Can you work these out from the model? Positions are in its coordinate system, mm. Face numbers are marked on the shaded views. A direction names the side the tool comes from. Coordinates: 2 decimals unless noted, no trailing zeros. Loops run counter-clockwise (first coordinate to the right, second up) from the corner with the lowest first, then second, coordinate; pieces in that order, holes last.
```python
from build123d import *

# Parameters (mm, degrees)
SKETCH2_W           = 80
SKETCH2_H           = 100
BOSS_EXTRUDE1_DEPTH = 10
SKETCH3_W           = 20
SKETCH3_H           = 100
BOSS_EXTRUDE2_DEPTH = 120
SKETCH5_R           = 2.555
CUT_EXTRUDE2_DEPTH  = 55
SKETCH4_R           = 15
CUT_EXTRUDE3_DEPTH  = 29


with BuildPart() as part:
    # Sketch2 → Boss-Extrude1 (new body)
    with BuildSketch(Plane(origin=(0, 0, 0), x_dir=(1, 0, 0), z_dir=(0, 1, 0))):
        Rectangle(SKETCH2_W, SKETCH2_H)
    extrude(amount=BOSS_EXTRUDE1_DEPTH)

    # Sketch3 → Boss-Extrude2 (add)
    with BuildSketch(Plane(origin=(0, 10, 0), x_dir=(1, 0, 0), z_dir=(0, 1, 0))):
        Rectangle(SKETCH3_W, SKETCH3_H)
    extrude(amount=BOSS_EXTRUDE2_DEPTH)

    # Sketch5 → Cut-Extrude2 (cut)
    with BuildSketch(Plane.XZ):
        with Locations((-25.4, -38.1)):
            Circle(SKETCH5_R)
        with Locations((25.4, -38.1)):
            Circle(SKETCH5_R)
        with Locations((-25.4, 38.1)):
            Circle(SKETCH5_R)
        with Locations((25.4, 38.1)):
            Circle(SKETCH5_R)
    extrude(amount=-CUT_EXTRUDE2_DEPTH, mode=Mode.SUBTRACT)

    # Sketch4 → Cut-Extrude3 (cut)
    with BuildSketch(Plane.ZY.offset(10)):
        with Locations((0, 103.69)):
            Circle(SKETCH4_R)
    extrude(amount=-CUT_EXTRUDE3_DEPTH, mode=Mode.SUBTRACT)


solid = part.part
```
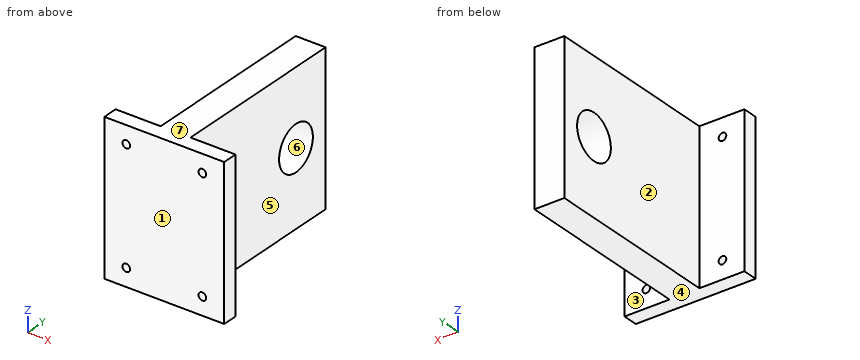
(1) I want a section at B-B on x = -25.4. Write out the boundary of the cut face in (y, z) (3 decimals).
Check values:
outline: (0, -50) - (10, -50) - (10, -40.655) - (0, -40.655) - close; (0, -35.545) - (10, -35.545) - (10, 35.545) - (0, 35.545) - close; (0, 40.655) - (10, 40.655) - (10, 50) - (0, 50) - close
(2) I want a section at A-A on z = -38.1. Write out the boundary of the cut face in (x, y) (3 decimals).
Check values:
outline: (-40, 0) - (-27.955, 0) - (-27.955, 10) - (-40, 10) - close; (-22.845, 0) - (22.845, 0) - (22.845, 10) - (10, 10) - (10, 130) - (-10, 130) - (-10, 10) - (-22.845, 10) - close; (27.955, 0) - (40, 0) - (40, 10) - (27.955, 10) - close
(3) If we mould it in two halves opening along Z, with no side actions, what happens to the marked faces 4, 5, 6 and 7? For each: released by +Z, released by -Z, zero draft, split by the parting line, or undercut.
Check values:
face 4: released by -Z
face 5: zero draft
face 6: undercut
face 7: released by +Z
(4) I want a section at D-D on z = 0. Write out the boundary of the cut face in (x, y), then the cut area to 3 significant figures.
Check values:
outline: (-40, 0) - (40, 0) - (40, 10) - (10, 10) - (10, 88.69) - (-10, 88.69) - (-10, 10) - (-40, 10) - close; (-10, 118.69) - (10, 118.69) - (10, 130) - (-10, 130) - close
area: 2,600 mm2
(5) If I drill on probe 1 along X at (y, z) = (3, -38); probe 2 along Z at (x, y) = (-3, 103); probe 3 along Y at (x, z) = (5.75, 0), over which ranges is the centre line in solid material (lowest first)?
Check values:
probe 1: x = -40 to -27.95, -22.85 to 22.85, 27.95 to 40
probe 2: z = -50 to -14.98, 14.98 to 50
probe 3: y = 0 to 88.69, 118.69 to 130
(6) Which directions (+Z, -Z, +X, -X, +Y, -Y) give clear straight access to the entire face, cutting with the end or side of a thin tool? Please do the marked faces 1, 2 and 3.
Check values:
face 1: +Z, -Z, +X, -X, -Y
face 2: +Z, -Z, -X, +Y
face 3: +Z, -Z, +X, +Y
(7) I want a section at C-C on y = 103.69. Write out the boundary of the cut face in (x, z).
Check values:
outline: (-10, -50) - (10, -50) - (10, -15) - (-10, -15) - close; (-10, 15) - (10, 15) - (10, 50) - (-10, 50) - close
(8) I'm going to push flat-ended pins straight in: pin 1 (9 mm diameter, centred on x = -18.5, z = -5.5, fed in from +Y); pin 2 (1.5 mm diameter, centred on y = 16, z = 3, fed in from -X). Where does each tip first touch, or does it pass through?
Check values:
pin 1: stops at y = 10
pin 2: stops at x = -10
